Work out the finished part from the listing and answer in its coordinate system (mm). Give positions to 0.01 mm unless a question says otherwise; leave off trailing zeros. Write each loop counter-clockwise with the first axis right and the second up, starting at its lowest first coordinate (ties: lowest second). Pieces come first, ordered by that corner, then holes. Notation, with made-up numbers: (-14, 25.5) -> (39, 25.5) arc R29 ccw to (39, 55.5) -> close; hole circle Ø3 at (16.25, 11.5). An arc over 180 degrees is marked (long way). Use a Markdown table: item, result. Add a question column.
Q1. Consider line 1 (X direction, y = 4.25, z = 0); line 2 (Z direction, x = 15.5, y = 4.25); line 3 (X direction, y = 3.75, z = -2.5). Determine where each line is inside the solid, lowest interval first.
Q2. Section D-D, the plane y = 1.25 is taken. Give the vertices of the cut face in (x, z) (3 decimals), plus the area to 3 significant figures.
Q3. This flat-tipped pin is pushed along its axis until it touches: pin 1 Ø4 at (x, z) = (-15.5, -15.5) entering from -Y. Where does it stop, or does it pass through?
Q4. For a pull along X with two mould halves and no side action, classify faces 1 (the face through (-32.9, 3.13, -14.25)), 2 (the face through (32.9, 3.13, -14.25)), 3 (the face through (-43.87, 3.13, 3.55)) as pulls with the +X half, pulls with the -X half, needs draft (parallel to the pull), parting line crosses it, or undercut.
Q5. Section B-B, the plane z = 0 is taken. Give the vertices of the cut face in (x, y), plus the area to 3 significant figures.
Q6. Section A-A, the plane x = 0 is taken. Give the vertices of the cut face in (y, z).
Q7. Section C-C, the plane x = -15.5 is taken. Give the vertices of the cut face in (y, z), plus the area to 3 significant figures.
Autodesk Inventor part; units mm, degrees
ref_plane "YZ Plane" through (0, 0, 0) normal (1, 0, 0) x (0, 1, 0)
ref_plane "XZ Plane" through (0, 0, 0) normal (0, 1, 0) x (-1, 0, 0)
ref_plane "XY Plane" through (0, 0, 0) normal (0, 0, 1) x (1, 0, 0)
sketch "Sketch1" plane through (0, 0, 0) normal (0, 1, 0) x (-1, 0, 0)
  line L0 (-21, -21) -> (21, -21)
  line L1 (21, -21) -> (21, 21)
  line L2 (21, 21) -> (-21, 21)
  line L3 (-21, 21) -> (-21, -21)
  line L4 (-21, -21) -> (21, 21) construction
  line L5 (21, -21) -> (-21, 21) construction
  circle A0 centre (15.5, 15.5) radius 1.75
  circle A1 centre (0, 0) radius 5.5
  line L6 (34.796, 0) -> (-29.6686, 0)
  line L7 (0, -38.1967) -> (0, 38.2612)
  circle A2 centre (15.5, -15.5) radius 1.75
  circle A3 centre (-15.5, 15.5) radius 1.75
  circle A4 centre (-15.5, -15.5) radius 1.75
  dimension "d0" = 42
  dimension "d1" = 42
  dimension "d4" = 3.5
  dimension "d8" = 11
  dimension "d13" = 31
extrude "Extrusion4" add sketch "Sketch1" along normal blind 6.35 contours L3 L6 A1 L7 L0 | L7 A1 L6 L1 L0 | L3 L2 L7 A1 L6 | L6 A1 L7 L2 L1
sketch "Sketch2" plane through (0, 0, 0) normal (0, -1, 0) x (1, 0, 0)
  line L0 (0, 45.4999) -> (0, -47.5937)
  line L1 (43.084, 0) -> (-45.3389, 0)
  arc A0 (-44.3867, 7.7323) -> (-44.3867, -7.7323) centre (-40, 0) ccw
  line L2 (-21, -21) -> (-21, 21)
  arc A1 (44.3867, -7.7323) -> (44.3867, 7.7323) centre (40, 0) ccw
  line L3 (-21, 21) -> (-21, -21)
  line L4 (-21, -21) -> (-21, 21)
  line L5 (21, 21) -> (21, -21)
  line L6 (21, 21) -> (21, -21)
  circle A2 centre (-40, 0) radius 5.25
  circle A3 centre (40, 0) radius 5.25
  line L7 (-21, -21) -> (-44.3867, -7.7323)
  line L8 (-44.3867, 7.7323) -> (-21, 21)
  line L9 (-21, 21) -> (-21, -21)
  line L10 (21, -21) -> (44.3867, -7.7323)
  line L11 (44.3867, 7.7323) -> (21, 21)
  point P0 (0, 0)
  dimension "d18" = 10.5
  dimension "d20" = 80
  dimension "d21" = 8.89
extrude "Extrusion5" add sketch "Sketch2" against normal up to surface (6.35 mm away)
fillet "Fillet1" radius 3.175 4 edges at (-21, 3.175, -21) (21, 3.175, -21) (21, 3.175, 21) (-21, 3.175, 21)
equation "\"d0\" = d1"
properties part number "Vertical_Lead_Screw_Shaft_Mount_Plate_Mid"
Result set:
| question | item | result |
|---|---|---|
| 1 | line 1 | x = -48.89 to -45.25, -34.75 to -5.5, 5.5 to 34.75, 45.25 to 48.89 |
| 1 | line 2 | z = -21 to -17.25, -13.75 to 13.75, 17.25 to 21 |
| 1 | line 3 | x = -48.53 to -44.62, -35.38 to -4.9, 4.9 to 35.38, 44.62 to 48.53 |
| 2 | outline | (-44.387, -7.732) -> (-21.729, -20.587) arc R3.175 ccw to (-20.162, -21) -> (20.162, -21) arc R3.175 ccw to (21.729, -20.587) -> (44.387, -7.732) arc R8.89 ccw to (44.387, 7.732) -> (21.729, 20.587) arc R3.175 ccw to (20.162, 21) -> (-20.162, 21) arc R3.175 ccw to (-21.729, 20.587) -> (-44.387, 7.732) arc R8.89 ccw to start; hole circle Ø10.5 at (-40, 0); hole circle Ø3.5 at (-15.5, -15.5); hole circle Ø3.5 at (-15.5, 15.5); hole circle Ø11 at (0, 0); hole circle Ø3.5 at (15.5, -15.5); hole circle Ø3.5 at (15.5, 15.5); hole circle Ø10.5 at (40, 0) |
| 2 | area | 2,900 mm2 |
| 3 | pin 1 | stops at y = 0 |
| 4 | face 1 | pulls with the -X half |
| 4 | face 2 | pulls with the +X half |
| 4 | face 3 | undercut |
| 5 | outline | (-48.89, 0) -> (-45.25, 0) -> (-45.25, 6.35) -> (-48.89, 6.35) -> close; (-34.75, 0) -> (-5.5, 0) -> (-5.5, 6.35) -> (-34.75, 6.35) -> close; (5.5, 0) -> (34.75, 0) -> (34.75, 6.35) -> (5.5, 6.35) -> close; (45.25, 0) -> (48.89, 0) -> (48.89, 6.35) -> (45.25, 6.35) -> close |
| 5 | area | 418 mm2 |
| 6 | outline | (0, -21) -> (6.35, -21) -> (6.35, -5.5) -> (0, -5.5) -> close; (0, 5.5) -> (6.35, 5.5) -> (6.35, 21) -> (0, 21) -> close |
| 7 | outline | (0, -21) -> (6.35, -21) -> (6.35, -17.25) -> (0, -17.25) -> close; (0, -13.75) -> (6.35, -13.75) -> (6.35, 13.75) -> (0, 13.75) -> close; (0, 17.25) -> (6.35, 17.25) -> (6.35, 21) -> (0, 21) -> close |
| 7 | area | 222 mm2 |
